Read the model definition and answer for the solid it produces. Units are mm, in the model's axes. Face numbers are marked on the shaded views. A direction names the side the tool comes from. Round coordinates to 2 decimals unless told otherwise and drop trailing zeros. Loops run counter-clockwise (first coordinate to the right, second up) from the corner with the lowest first, then second, coordinate; pieces in that order, holes last. Notation, with made-up numbers: (-11, 78) - (42, 78) arc R13 cw to (42, 93) - close; hole circle Ø3 at (16, 85.5). An arc over 180 degrees is marked (long way). Use CSV: the item, a comma, the result in double quotes. Start each with the question number.
1. Given pin 1 Ø6.5 at (x, y) = (27.5, -5) entering from +Z; pin 2 Ø5.5 at (y, z) = (-4, 32.5) entering from +X; pin 3 Ø3.5 at (y, z) = (-10.5, 4.5) entering from +X; pin 4 Ø1 at (y, z) = (-2.5, 17.5) entering from -X, each flat-ended and moving along its own axis, determine where each tip first touches the part or whether it passes through.
2. Find section B-B (z = 32.5). Give the vertices of the cut face in (x, y).
3. A tool of negligible diameter and unlimited length cuts with its end or side. For the marked faces 1, 2, 3, 4 and 5, from which of +Z, -Z, +X, -X, +Y, -Y can it reach the whole face along a straight path? Write none if from no direction.
4. Find section C-C (x = 4). Give the vertices of the cut face in (y, z), and give its area (3 significant figures).
5. Find section A-A (y = -13). Give the vertices of the cut face in (x, z).
6. Consider line 1 along Y through (x, z) = (16, 2.7); line 2 along Y through (x, z) = (65.5, 32.5); line 3 along X through (y, z) = (-3, 12). Determine where each line is inside the solid, lowest interval first.
7. Find section D-D (y = -4). Give the vertices of the cut face in (x, z).
from build123d import *

# Parameters (mm, degrees)
BOSS_EXTRUDE1_DEPTH = 8
SKETCH2_W           = 6
SKETCH2_H           = 9
BOSS_EXTRUDE2_DEPTH = 20
CUT_EXTRUDE1_REACH  = 71.239
SKETCH3_R           = 3
SKETCH4_R           = 2
CUT_EXTRUDE2_DEPTH  = 10


with BuildPart() as part:
    # Sketch1 → Boss-Extrude1 (new body)
    with BuildSketch(Plane(origin=(0, 0, 0), x_dir=(1, 0, 0), z_dir=(0, 1, 0))):
        Polygon((0, 0), (0, -28), (56, -28), (56, -37), (70, -37), (70, -21), (30, -21), (20, -11), (20, 0), align=None)
    extrude(amount=-BOSS_EXTRUDE1_DEPTH)

    # Sketch2 → Boss-Extrude2 (add)
    with BuildSketch(Plane.ZY):
        with Locations((3, -12.5)):
            Rectangle(SKETCH2_W, SKETCH2_H)
    extrude(amount=-BOSS_EXTRUDE2_DEPTH)

    # Sketch3 → Cut-Extrude1 (cut, up to next)
    with BuildSketch(Plane.ZY.offset(-56), mode=Mode.PRIVATE) as cut_extrude1_sk1:
        with Locations((32.5, -4)):
            Circle(SKETCH3_R)
    cut_extrude1_tool1 = extrude(cut_extrude1_sk1.sketch, amount=-CUT_EXTRUDE1_REACH, mode=Mode.PRIVATE) & part.part
    add(cut_extrude1_tool1.solids().sort_by_distance((56, -4, 32.5))[0], mode=Mode.SUBTRACT)

    # Sketch4 → Cut-Extrude2 (cut)
    with BuildSketch(Plane.XY.offset(6)):
        with Locations((4, -13)):
            Circle(SKETCH4_R)
        with Locations((16, -13)):
            Circle(SKETCH4_R)
    extrude(amount=-CUT_EXTRUDE2_DEPTH, mode=Mode.SUBTRACT)


solid = part.part
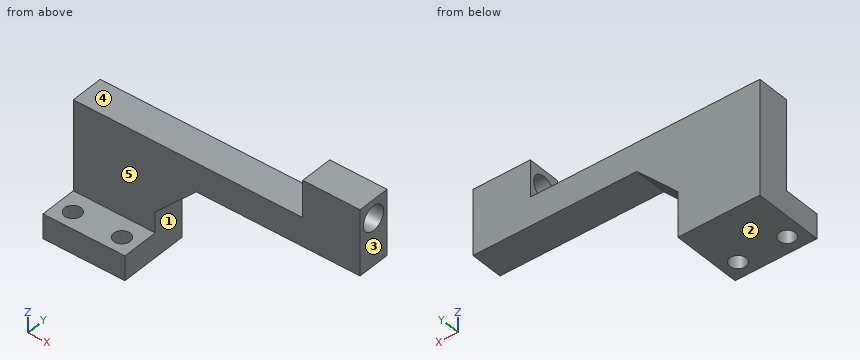
Filled sheet:
1,pin 1,"stops at z = 28"
1,pin 2,"passes through"
1,pin 3,"stops at x = 20"
1,pin 4,"stops at x = 0"
2,outline,"(56, -8) - (70, -8) - (70, -7) - (56, -7) - close; (56, -1) - (70, -1) - (70, 0) - (56, 0) - close"
3,face 1,"-Z, +X, +Y, -Y"
3,face 2,"-Z, +X, -X, +Y, -Y"
3,face 3,"+Z, -Z, +X, +Y, -Y"
3,face 4,"+Z, -X, +Y, -Y"
3,face 5,"+Z, +X, -X, -Y"
4,outline,"(-17, 0) - (-15, 0) - (-15, 6) - (-17, 6) - close; (-11, 0) - (0, 0) - (0, 28) - (-8, 28) - (-8, 6) - (-11, 6) - close"
4,area,"254 mm²"
5,outline,"(0, 0) - (2, 0) - (2, 6) - (0, 6) - close; (6, 0) - (14, 0) - (14, 6) - (6, 6) - close; (18, 0) - (20, 0) - (20, 6) - (18, 6) - close"
6,line 1,"y = -17 to -15, -11 to 0"
6,line 2,"y = -8 to -7, -1 to 0"
6,line 3,"x = 0 to 21"
7,outline,"(0, 0) - (20, 0) - (20, 11) - (30, 21) - (70, 21) - (70, 29.5) - (56, 29.5) - (56, 28) - (0, 28) - close; (56, 35.5) - (70, 35.5) - (70, 37) - (56, 37) - close"
